from build123d import *

# Parameters (mm, degrees)
BOSS_EXTRUDE1_DEPTH = 2.8
SKETCH2_W           = 22.2
SKETCH2_H           = 5
BOSS_EXTRUDE2_DEPTH = 2.8


with BuildPart() as part:
    # Sketch1 → Boss-Extrude1 (new body)
    with BuildSketch(Plane.XY):
        Polygon((30, 13.5), (30, 23.5), (-32.5, 23.5), (-32.5, -23.5), (30, -23.5), (30, -13.5), (-25, -13.5), (-25, 13.5), align=None)
    extrude(amount=BOSS_EXTRUDE1_DEPTH)

    # Sketch2 → Boss-Extrude2 (add)
    with BuildSketch(Plane(origin=(-30, 0, 0), x_dir=(0, 0, -1), z_dir=(1, 0, 0))):
        with BuildLine():
            Line((-2.8, -7.5), (-2.8, 7.5))
            Line((-2.8, 7.5), (-50, 7.5))
            ThreePointArc((-50, 7.5), (-57.5, 0), (-50, -7.5))
            Line((-50, -7.5), (-2.8, -7.5))
        make_face()
        with BuildLine():
            Line((-50, -2.5), (-37.5, -2.5))
            ThreePointArc((-37.5, -2.5), (-35, 0), (-37.5, 2.5))
            Line((-37.5, 2.5), (-50, 2.5))
            ThreePointArc((-50, 2.5), (-52.5, 0), (-50, -2.5))
        make_face(mode=Mode.SUBTRACT)
        with Locations((-18.9, 0)):
            Rectangle(SKETCH2_W, SKETCH2_H, mode=Mode.SUBTRACT)
    extrude(amount=BOSS_EXTRUDE2_DEPTH)


solid = part.part
For this review, take the finished solid that the model builds, in its own axes (mm). A direction names the side the tool comes from. Give positions to 0.01 mm unless a question says otherwise; leave off trailing zeros. Order: outer loops, then holes, each group sorted by start corner. A loop starts at its lowest first (then second) coordinate and runs counter-clockwise, first axis right, second up. Notation, with made-up numbers: M -29.75,-17 L -16.75,-17 A28 ccw -16.75,17 Z; hole C -25,-10 d10. An arc over 180 degrees is marked long. Answer in a Markdown table with one row per item. Add a question column.
(1) For faces 4 (the face through (-2, -23.5, 1)), 5 (the face through (-28.6, 0.1, 52.5)), 6 (the face through (-30, 0, 31)), 7 (the face through (3, -13.5, 1)), 8 (the face through (-27.2, 0, 31)), list the 3-axis set-ups (+Z, -Z, +X, -X, +Y, -Y) from which the entire face can be reached by the end or side of a thin tool; tool diameter is ignored.
(2) Consider section B-B on x = -10. State the section outline as (y, z) points.
(3) Wall thickness on probe 1 along X at (y, z) = (-5, 46); probe 2 along Z at (x, y) = (-9, -15); probe 3 along Y at (x, z) = (-29, 19): over which ranges is each line inside the solid? List them lowest first. Write a range as [from, to].
(4) Consider section A-A on y = 0. State the section outline as (x, z) points, and give its area (3 significant figures).
(5) For pin 1 (0.8 mm diameter, centred on y = -0.5, z = 1.5, fed in from +X); pin 2 (4.5 mm diameter, centred on y = 2, z = 29, fed in from -X); pin 3 (0.8 mm diameter, centred on x = -28.5, z = 44, fed in from +Y), all flat-tipped, find the tip position at first contact; note any pin that passes through.
(6) Mouldability with a two-part tool opening along Y and no side actions: class faces 1 (the face through (-29, -7.5, 27)), 2 (the face through (-32.5, 0, 1)), 3 (the face through (2, 13.5, 1)) as +Y half, -Y half, draft (parallel to the pull), parting line (faces both ways), or undercut.
(7) Consider section D-D on x = -29. State the section outline as (y, z) points.
(8) Consider section C-C on z = 40.5. State the section outline as (x, y) points, and give its area (3 significant figures).
Evaluation:
| question | item | result |
|---|---|---|
| 1 | face 4 | +Z, -Z, +X, -X, -Y |
| 1 | face 5 | +X, -X |
| 1 | face 6 | +Z, -X, +Y, -Y |
| 1 | face 7 | +Z, -Z, +X |
| 1 | face 8 | +Z, +X, +Y, -Y |
| 2 | outline | M -23.5,0 L -13.5,0 L -13.5,2.8 L -23.5,2.8 Z; M 13.5,0 L 23.5,0 L 23.5,2.8 L 13.5,2.8 Z |
| 3 | probe 1 | x = [-30, -27.2] |
| 3 | probe 2 | z = [0, 2.8] |
| 3 | probe 3 | y = [-7.5, -2.5], [2.5, 7.5] |
| 4 | outline | M -32.5,0 L -25,0 L -25,2.8 L -27.2,2.8 L -27.2,7.8 L -30,7.8 L -30,2.8 L -32.5,2.8 Z; M -30,30 L -27.2,30 L -27.2,35 L -30,35 Z; M -30,52.5 L -27.2,52.5 L -27.2,57.5 L -30,57.5 Z |
| 4 | area | 63.0 mm^2 |
| 5 | pin 1 | stops at x = -25 |
| 5 | pin 2 | stops at x = -30 |
| 5 | pin 3 | stops at y = 7.5 |
| 6 | face 1 | -Y half |
| 6 | face 2 | draft |
| 6 | face 3 | undercut |
| 7 | outline | M -23.5,0 L 23.5,0 L 23.5,2.8 L 7.5,2.8 L 7.5,50 A7.5 ccw -7.5,50 L -7.5,2.8 L -23.5,2.8 Z; hole M -2.5,7.8 L 2.5,7.8 L 2.5,30 L -2.5,30 Z; hole M -2.5,37.5 A2.5 ccw 2.5,37.5 L 2.5,50 A2.5 ccw -2.5,50 Z |
| 8 | outline | M -30,-7.5 L -27.2,-7.5 L -27.2,-2.5 L -30,-2.5 Z; M -30,2.5 L -27.2,2.5 L -27.2,7.5 L -30,7.5 Z |
| 8 | area | 28.0 mm^2 |
